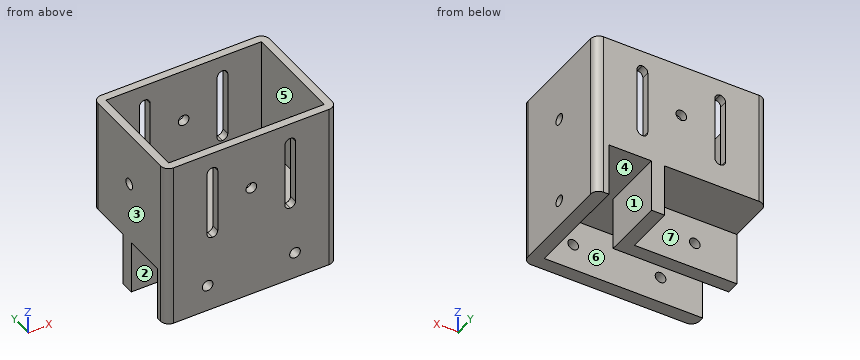
from build123d import *

# Parameters (mm, degrees)
F0_W          = 64.5
F0_H          = 44.5
F0_W_2        = 58.5
F0_H_2        = 38.5
F1_DEPTH      = 40
F2_DEPTH      = 3
F4_DEPTH      = 20
F5_R          = 2
F6_DEPTH      = 3.001
F6_DEPTH_BACK = 41.5
F7_R          = 3
F8_R          = 2
F9_DEPTH      = 25
F10_R         = 2
F11_DEPTH     = 25
F12_R         = 2
F13_DEPTH     = 64.501


with BuildPart() as f1:
    # F0 (on Top) → F1 (new body)
    with BuildSketch(Plane.XY):
        Rectangle(F0_W, F0_H)
        Rectangle(F0_W_2, F0_H_2, mode=Mode.SUBTRACT)
    extrude(amount=F1_DEPTH)

    # F0 (on Top) → F2 (join)
    with BuildSketch(Plane.XY):
        Rectangle(F0_W, F0_H)
        Rectangle(F0_W_2, F0_H_2, mode=Mode.SUBTRACT)
        Rectangle(F0_W_2, F0_H_2)
    extrude(amount=-F2_DEPTH)

    # F3 (on face) → F4 (join)
    with BuildSketch(Plane(origin=(0, 0, -3), x_dir=(1, 0, 0), z_dir=(0, 0, -1))):
        Polygon((27.25, -22.25), (32.25, -22.25), (32.25, 22.25), (-32.25, 22.25), (-32.25, 17.25), (27.25, 17.25), align=None)
        Polygon((11.25, 1.25), (-32.25, 1.25), (-32.25, -3.75), (6.25, -3.75), (6.25, -22.25), (11.25, -22.25), align=None)
    extrude(amount=F4_DEPTH)

    # F5 (on face) → F6 (cut, two sides)
    with BuildSketch(Plane.XZ.offset(-19.25)) as f6_sk:
        with BuildLine():
            ThreePointArc((14.625, 5.8733418593), (16.0392135624, 6.4591282969), (16.625, 7.8733418593))
            Line((16.625, 7.8733418593), (16.625, 32.1266581407))
            ThreePointArc((16.625, 32.1266581407), (16.0392135624, 33.5408717031), (14.625, 34.1266581407))
            ThreePointArc((14.625, 34.1266581407), (13.2107864376, 33.5408717031), (12.625, 32.1266581407))
            Line((12.625, 32.1266581407), (12.625, 7.8733418593))
            ThreePointArc((12.625, 7.8733418593), (13.2107864376, 6.4591282969), (14.625, 5.8733418593))
        make_face()
        with BuildLine():
            ThreePointArc((-12.625, 32.1266581407), (-13.2107864376, 33.5408717031), (-14.625, 34.1266581407))
            ThreePointArc((-14.625, 34.1266581407), (-16.0392135624, 33.5408717031), (-16.625, 32.1266581407))
            Line((-16.625, 32.1266581407), (-16.625, 7.8733418593))
            ThreePointArc((-16.625, 7.8733418593), (-16.0392135624, 6.4591282969), (-14.625, 5.8733418593))
            ThreePointArc((-14.625, 5.8733418593), (-13.2107864376, 6.4591282969), (-12.625, 7.8733418593))
            Line((-12.625, 7.8733418593), (-12.625, 32.1266581407))
        make_face()
        with Locations((0, 20)):
            Circle(F5_R)
    extrude(amount=-F6_DEPTH, mode=Mode.SUBTRACT)
    extrude(f6_sk.sketch, amount=F6_DEPTH_BACK, mode=Mode.SUBTRACT)

    # F7
    f7_edges = [f1.edges().sort_by_distance(p)[0] for p in [
        (-32.25, 22.25, 18.5),
        (-32.25, -22.25, 8.5),
        (32.25, 22.25, 8.5),
        (32.25, -22.25, 8.5),
    ]]
    fillet(f7_edges, radius=F7_R)

    # F8 (on face) → F9 (cut, symmetric)
    with BuildSketch(Plane(origin=(0, -17.25, 0), x_dir=(-1, 0, 0), z_dir=(0, 1, 0))):
        with Locations((16.4400730282, -13)):
            Circle(F8_R)
        with Locations((-16.4400730282, -13)):
            Circle(F8_R)
    extrude(amount=F9_DEPTH, both=True, mode=Mode.SUBTRACT)

    # F10 (on face) → F11 (cut)
    with BuildSketch(Plane(origin=(27.25, 0, 0), x_dir=(0, -1, 0), z_dir=(-1, 0, 0))):
        with Locations((0, -13)):
            Circle(F10_R)
    extrude(amount=-F11_DEPTH, mode=Mode.SUBTRACT)

    # F12 (on face) → F13 (cut, through all)
    with BuildSketch(Plane(origin=(-32.25, 0, 0), x_dir=(0, -1, 0), z_dir=(-1, 0, 0))):
        with Locations((0, 20)):
            Circle(F12_R)
    extrude(amount=-F13_DEPTH, mode=Mode.SUBTRACT)


solid = f1.part
Input: part model. Units: mm. Frame: model coordinates. Face numbers are marked on the shaded views. A direction names the side the tool comes from. Give positions to 0.01 mm unless a question says otherwise; leave off trailing zeros. Write each loop counter-clockwise with the first axis right and the second up, starting at its lowest first coordinate (ties: lowest second). Pieces come first, ordered by that corner, then holes. Notation, with made-up numbers: M 88,24 L 147,24 A36 ccw 147,60 Z; hole C 86,56 d5. An arc over 180 degrees is marked long. Use one line per item in the form item = value.
1. Mould query, pull axis X, two halves, no side actions, for the marked faces 1, 2, 3 and 4. Classes: released by +X, released by -X, zero draft, split by the parting line, or undercut.
Outcome:
face_1 = undercut
face_2 = zero draft
face_3 = released by -X
face_4 = undercut
2. Cut plane D-D on y = -10.5. Return loops of the section in (x, z).
Outcome:
outline = M -32.25,-3 L 27.25,-3 L 27.25,-23 L 32.25,-23 L 32.25,40 L 29.25,40 L 29.25,0 L -29.25,0 L -29.25,40 L -32.25,40 Z
3. First-contact query: P1, Ø5, axis at x = -0.5, y = 5.5, coming from the -Z side; P2, Ø3, axis at x = -11, y = -12, coming from the -Z side; P3, Ø2.5, axis at y = 21.5, z = 19, coming from the -X side; P4, Ø0.9, axis at y = -20, z = 23, coming from the -X side. Flat tips, straight axial feed; report the tip coordinate or a pass-through.
Outcome:
P1 = -23
P2 = -3
P3 = -32.08
P4 = -32.23
4. Cut plane A-A on y = 0. Return loops of the section in (x, z), and give its area (3 significant figures).
Outcome:
outline = M -32.25,-23 L 11.25,-23 L 11.25,-3 L 27.25,-3 L 27.25,-11 L 32.25,-11 L 32.25,18 L 29.25,18 L 29.25,0 L -29.25,0 L -29.25,18 L -32.25,18 Z; M -32.25,22 L -29.25,22 L -29.25,40 L -32.25,40 Z; M 27.25,-23 L 32.25,-23 L 32.25,-15 L 27.25,-15 Z; M 29.25,22 L 32.25,22 L 32.25,40 L 29.25,40 Z; hole C -16.44,-13 d4
area = 1,350 mm²
5. Ray query, L1, parallel to Z at x = 30.2, y = 0; L2, parallel to X at y = -19.5, z = 25 (3 decimals); L3, parallel to Y at x = 23.5, z = 32.5. Return the intervals inside material, ascending.
Outcome:
L1 = -23 to -15, -11 to 18, 22 to 40
L2 = -32.24 to -16.625, -12.625 to 12.625, 16.625 to 32.24
L3 = -22.25 to -19.25, 19.25 to 22.25
6. Cut plane C-C on z = -13. State how many separate pieces and enclosed holes the cut face has, and give its area (3 significant figures).
Outcome:
separate_pieces = 6
enclosed_holes = 0
area = 744 mm²
7. Reachability of the marked faces 5, 6 and 7 from +Z, -Z, +X, -X, +Y, -Y: full face, straight path, thin tool, end or side. Return the list, or none.
Outcome:
face_5 = +Z
face_6 = -Z, -X
face_7 = -Z, -X, +Y
8. Cut plane B-B on x = 0. Return loops of the section in (y, z).
Outcome:
outline = M -22.25,-23 L -17.25,-23 L -17.25,-3 L -1.25,-3 L -1.25,-23 L 3.75,-23 L 3.75,-3 L 22.25,-3 L 22.25,18 L 19.25,18 L 19.25,0 L -19.25,0 L -19.25,18 L -22.25,18 Z; M -22.25,22 L -19.25,22 L -19.25,40 L -22.25,40 Z; M 19.25,22 L 22.25,22 L 22.25,40 L 19.25,40 Z
